Check sheet for the drawn part. Datum: minimum x, y, z corner. Units: mm. Round coordinates to 2 decimals unless told otherwise and drop trailing zeros. Write each loop counter-clockwise with the first axis right and the second up, starting at its lowest first coordinate (ties: lowest second). Pieces come first, ordered by that corner, then holes.
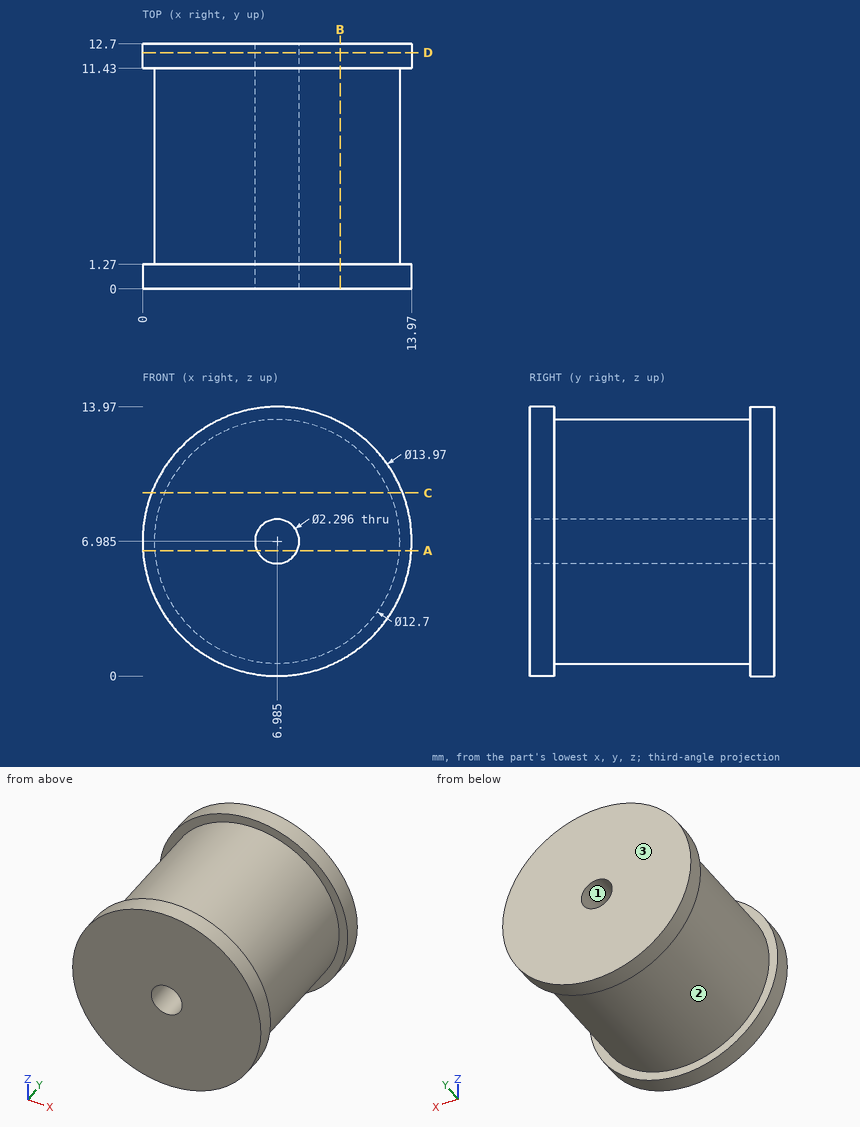
Q1. Material ranges on line 1 along Y through (x, z) = (5, 13.25); line 2 along X through (y, z) = (9.5, 7.5); line 3 along Z through (x, y) = (7, 12.25), recorded low to high.
Recorded:
line 1: y = 0 to 1.27, 11.43 to 12.7
line 2: x = 0.66 to 5.96, 8.01 to 13.31
line 3: z = 0 to 5.84, 8.13 to 13.97
Q2. Release check for a two-part mould opening along Z. For the marked faces 1, 2 and 3 record: released by +Z, released by -Z, zero draft, split by the parting line, or undercut.
Recorded:
face 1: undercut
face 2: split by the parting line
face 3: zero draft
Q3. Sectioned sample at D-D (y = 12.25). Enter the section's corners in (x, z) (3 decimals).
Recorded:
outline: circle Ø13.97 at (6.985, 6.985); hole circle Ø2.296 at (6.985, 6.985)
Q4. Sectioned sample at B-B (x = 10.25). Enter the section's corners in (y, z).
Recorded:
outline: (0, 0.81) - (1.27, 0.81) - (1.27, 1.54) - (11.43, 1.54) - (11.43, 0.81) - (12.7, 0.81) - (12.7, 13.16) - (11.43, 13.16) - (11.43, 12.43) - (1.27, 12.43) - (1.27, 13.16) - (0, 13.16) - close
Q5. Depth check by flat-ended pin: P1, Ø2, axis at y = 6, z = 10.5, coming from the -X side; P2, Ø1, axis at y = 10.5, z = 11, coming from the +X side; P3, Ø4, axis at x = 10.5, z = 7.5, coming from the -Y side; P4, Ø2, axis at x = 9, y = 10, coming from the +Z side. Enter the tip coordinate at first touch or a pass-through.
Recorded:
P1: stops at x = 1.15
P2: stops at x = 12.27
P3: stops at y = 0
P4: stops at z = 13.25
Q6. Sectioned sample at A-A (z = 6.5). Enter the section's corners in (x, y).
Recorded:
outline: (0.02, 0) - (5.94, 0) - (5.94, 12.7) - (0.02, 12.7) - (0.02, 11.43) - (0.65, 11.43) - (0.65, 1.27) - (0.02, 1.27) - close; (8.03, 0) - (13.95, 0) - (13.95, 1.27) - (13.32, 1.27) - (13.32, 11.43) - (13.95, 11.43) - (13.95, 12.7) - (8.03, 12.7) - close
Q7. Sectioned sample at C-C (z = 9.5). Enter the section's corners in (x, y), plus the area to 3 significant figures.
Recorded:
outline: (0.47, 0) - (13.5, 0) - (13.5, 1.27) - (12.82, 1.27) - (12.82, 11.43) - (13.5, 11.43) - (13.5, 12.7) - (0.47, 12.7) - (0.47, 11.43) - (1.15, 11.43) - (1.15, 1.27) - (0.47, 1.27) - close
area: 152 mm2
